Geometry: see drawing. Coordinates: mm, zero at the bounding-box minimum. A direction names the side the tool comes from. Coordinates: 2 decimals unless noted, no trailing zeros. Write each loop counter-clockwise with the first axis right and the second up, starting at its lowest first coordinate (ties: lowest second). Pieces come first, ordered by that corner, then holes. Notation, with made-up numbers: (3, -30.5) -> (41, -30.5) arc R8 ccw to (41, -22.5) -> close; hole circle Ø6 at (-12, 58.5). An arc over 180 degrees is marked (long way). Use one line per item in the form item = value. Start each with the question number.
(1) Cut plane A-A on z = 5. Return the cut outline in (x, y).
(2) Ray query, line 1 along Z through (x, y) = (88.5, 9.25); line 2 along Y through (x, z) = (77, 15.75). Return the intervals inside material, ascending.
(3) Cut plane D-D on x = 96.5. Return the cut outline in (y, z).
(4) Set-up query: the marked faces 1 and 2. Return all of +Z, -Z, +X, -X, +Y, -Y with unobstructed straight access to the full face (end or side cutting, diameter ignored); none if empty.
(5) Cut plane C-C on y = 16.5. Return the cut outline in (x, z).
(6) First-contact query: pin 1 (7 mm diameter, centred on x = 94.5, z = 15, fed in from +Y); pin 2 (11.5 mm diameter, centred on x = 115, y = 11, fed in from -Z). Flat tips, straight axial feed; report the tip coordinate or a pass-through.
(7) Cut plane B-B on x = 34.5. Return the cut outline in (y, z).
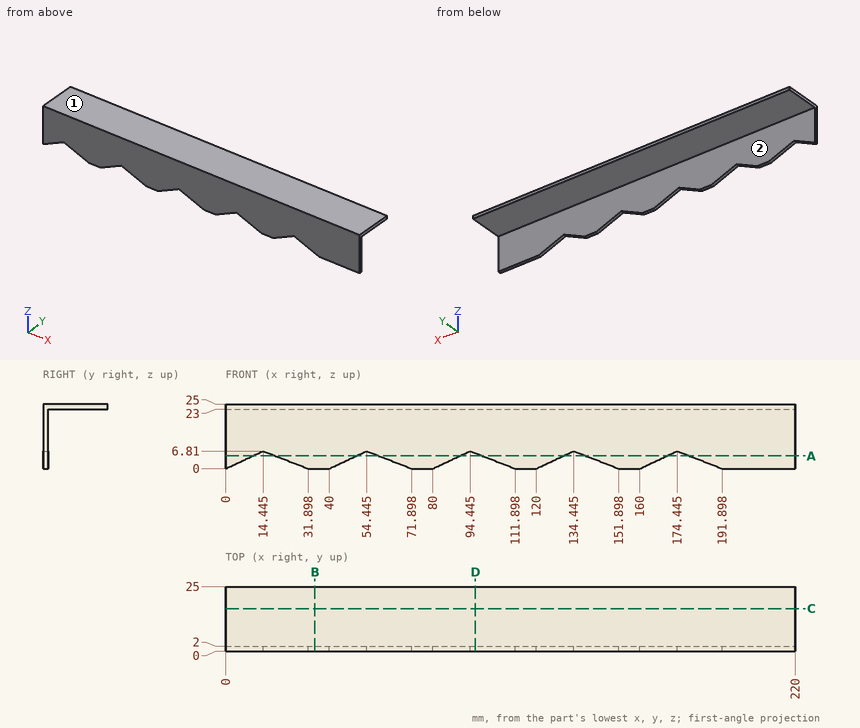
Values:
q1.outline = (0, 0) -> (10.61, 0) -> (10.61, 2) -> (0, 2) -> close; (19.08, 0) -> (50.61, 0) -> (50.61, 2) -> (19.08, 2) -> close; (59.08, 0) -> (90.61, 0) -> (90.61, 2) -> (59.08, 2) -> close; (99.08, 0) -> (130.61, 0) -> (130.61, 2) -> (99.08, 2) -> close; (139.08, 0) -> (170.61, 0) -> (170.61, 2) -> (139.08, 2) -> close; (179.08, 0) -> (220, 0) -> (220, 2) -> (179.08, 2) -> close
q2.line_1 = 23 to 25
q2.line_2 = 0 to 2
q3.outline = (0, 6.01) -> (2, 6.01) -> (2, 23) -> (25, 23) -> (25, 25) -> (0, 25) -> close
q4.face_1 = +Z, +X, -X, +Y, -Y
q4.face_2 = -Z, +X, -X, +Y
q5.outline = (0, 23) -> (220, 23) -> (220, 25) -> (0, 25) -> close
q6.pin_1 = 2
q6.pin_2 = 23
q7.outline = (0, 0) -> (2, 0) -> (2, 23) -> (25, 23) -> (25, 25) -> (0, 25) -> close
